Job drawing, mm, ordinate dimensions from the low corner. One solid piece. A direction names the side the tool comes from. Round coordinates to 2 decimals unless told otherwise and drop trailing zeros. Loops run counter-clockwise (first coordinate to the right, second up) from the corner with the lowest first, then second, coordinate; pieces in that order, holes last.
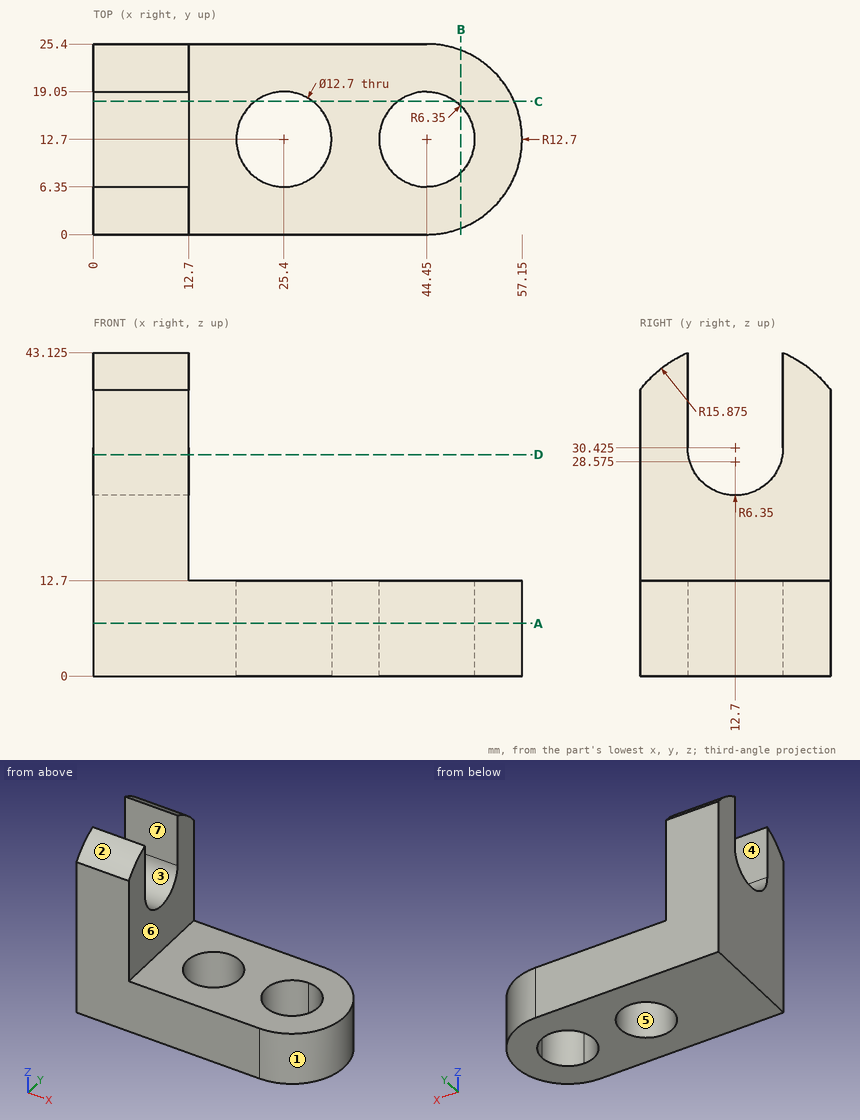
(1) Which spindle directions (+Z, -Z, +X, -X, +Y, -Y) get a long thin tool onto all of the face, cutting with end or side? Do the marked faces 5, 6 and 7. Say none if no direction does.
Responses:
face 5: +Z, -Z
face 6: +Z, +X, +Y, -Y
face 7: +Z, +X, -X
(2) Slice it at C-C on y = 17.75. Count the separate pieces of the cut face and the enclosed holes in it, plus the area to 3 significant figures.
Responses:
separate pieces: 3
enclosed holes: 0
area: 693 mm2
(3) Pin check, flat tips, straight feed: P1, Ø1.5, axis at y = 10, z = 28, coming from the -X side; P2, Ø12, axis at y = 9, z = 33.5, coming from the +X side; P3, Ø7.5, axis at x = 44, y = 15.5, coming from the +Z side. Stop position of each tip, or through.
Responses:
P1: passes through
P2: stops at x = 12.7
P3: stops at z = 12.7
(4) Probe line 1 (Y direction, x = 25.4, z = 6); line 2 (X direction, y = 9, z = 6); line 3 (Z direction, x = 26, y = 5). List the from-to ranges inside material, lowest first.
Responses:
line 1: y = 0 to 6.35, 19.05 to 25.4
line 2: x = 0 to 20.24, 30.56 to 39.29, 49.61 to 56.6
line 3: z = 0 to 12.7
(5) Slice it at A-A on z = 7. List the corners of the cut face in (x, y).
Responses:
outline: (0, 0) - (44.45, 0) arc R12.7 ccw to (44.45, 25.4) - (0, 25.4) - close; hole circle Ø12.7 at (25.4, 12.7); hole circle Ø12.7 at (44.45, 12.7)
(6) Slice it at D-D on z = 29.5. List the corners of the cut face in (x, y), plus the area to 3 significant figures.
Responses:
outline: (0, 0) - (12.7, 0) - (12.7, 6.42) - (0, 6.42) - close; (0, 18.98) - (12.7, 18.98) - (12.7, 25.4) - (0, 25.4) - close
area: 163 mm2
(7) Slice it at B-B on x = 49. List the corners of the cut face in (y, z).
Responses:
outline: (0.84, 0) - (8.27, 0) - (8.27, 12.7) - (0.84, 12.7) - close; (17.13, 0) - (24.56, 0) - (24.56, 12.7) - (17.13, 12.7) - close
(8) Pull direction Y, two halves, no side cores. Call the marked faces 1, 2, 3 and 4: +Y half, -Y half, draft (parallel to the pull), parting line (faces both ways), or undercut.
Responses:
face 1: parting line
face 2: -Y half
face 3: undercut
face 4: undercut
